```python
from build123d import *

# Parameters (mm, degrees)
SKETCH1_W                    = 25.4
SKETCH1_H                    = 25.4
SKETCH1_W_2                  = 22.225
SKETCH1_H_2                  = 22.225
BOSS_EXTRUDE1_DEPTH          = 863.6
F_1_4_0_25_DIAMETER_HOLE1_D  = 6.35
F_3_8_0_375_DIAMETER_HOLE1_D = 9.525
F_5_8_0_625_DIAMETER_HOLE1_D = 15.875
F_1_4_0_25_DIAMETER_HOLE2_D  = 6.35


with BuildPart() as part:
    # Sketch1 → Boss-Extrude1 (new body)
    with BuildSketch(Plane(origin=(0, 0, 0), x_dir=(1, 0, 0), z_dir=(0, 1, 0))):
        Rectangle(SKETCH1_W, SKETCH1_H)
        Rectangle(SKETCH1_W_2, SKETCH1_H_2, mode=Mode.SUBTRACT)
    extrude(amount=BOSS_EXTRUDE1_DEPTH)

    # 1/4 (0.25) Diameter Hole1 (through all)
    with Locations(Plane(origin=(12.7, 0, 0), x_dir=(0, 0, -1), z_dir=(1, 0, 0))):
        with Locations((0, 177.8), (0, 850.9), (0, 15.398282467), (0, 431.8), (0, 558.8), (0, 685.8), (0, 304.8)):
            Hole(F_1_4_0_25_DIAMETER_HOLE1_D / 2)

    # 3/8 (0.375) Diameter Hole1 (through all)
    with Locations(Plane(origin=(12.7, 0, 0), x_dir=(0, 0, -1), z_dir=(1, 0, 0))):
        with Locations((0, 48.900570065), (0, 818.04497499)):
            Hole(F_3_8_0_375_DIAMETER_HOLE1_D / 2)

    # 5/8 (0.625) Diameter Hole1 (through all)
    with Locations(Plane(origin=(12.7, 0, 0), x_dir=(0, 0, -1), z_dir=(1, 0, 0))):
        with Locations((0, 737.710800359)):
            Hole(F_5_8_0_625_DIAMETER_HOLE1_D / 2)

    # 1/4 (0.25) Diameter Hole2 (through all)
    with Locations(Plane(origin=(12.7, 0, 0), x_dir=(0, 0, -1), z_dir=(1, 0, 0))):
        with Locations((0, 712.310800359), (0, 763.110800359)):
            Hole(F_1_4_0_25_DIAMETER_HOLE2_D / 2)


solid = part.part
```
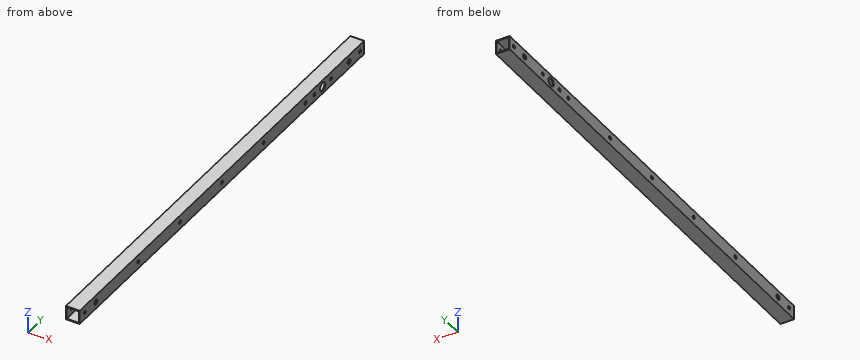
Build history of the part. All positions in model axes, mm. Give positions to 0.01 mm unless a question says otherwise; leave off trailing zeros. Loops run counter-clockwise (first coordinate to the right, second up) from the corner with the lowest first, then second, coordinate; pieces in that order, holes last.
1) Probe line 1 along X through (y, z) = (709, -9); line 2 along Z through (x, y) = (11.5, 685.8) (3 decimals). List the from-to ranges inside material, lowest first.
Values follow:
line 1: x = -12.7 to -11.11, 11.11 to 12.7
line 2: z = -12.7 to -3.175, 3.175 to 12.7
2) Band-saw the part on A-A on x = 3.25. List the corners of the cut face in (y, z).
Values follow:
outline: (0, -12.7) - (863.6, -12.7) - (863.6, -11.11) - (0, -11.11) - close; (0, 11.11) - (863.6, 11.11) - (863.6, 12.7) - (0, 12.7) - close
3) Drop a flat-ended pin along its axis: P1, Ø5.5, axis at y = 15.4, z = 0, coming from the -X side. Give the stop position or say it passes through.
Values follow:
P1: passes through
4) Band-saw the part on B-B on y = 580.5. List the corners of the cut face in (x, z).
Values follow:
outline: (-12.7, -12.7) - (12.7, -12.7) - (12.7, 12.7) - (-12.7, 12.7) - close; hole (-11.11, -11.11) - (11.11, -11.11) - (11.11, 11.11) - (-11.11, 11.11) - close
